The model under review builds one solid part; all positions refer to its coordinate system, in mm. A direction names the side the tool comes from. Coordinates: 2 decimals unless noted, no trailing zeros. Loops run counter-clockwise (first coordinate to the right, second up) from the corner with the lowest first, then second, coordinate; pieces in that order, holes last. Notation, with made-up numbers: (79, 12.5) - (103, 12.5) arc R5 cw to (103, 21.5) - close; hole circle Ø7 at (-33.5, -10). An arc over 180 degrees is marked (long way). One line per item, written item: value. Start each with the question number.
1. To check wall thickness, follow line 1 (Z direction, x = -60.75, y = 7.5); line 2 (X direction, y = 1.5, z = 12.75); line 3 (Z direction, x = -57, y = 10). State the ranges of each line that lie inside material, in increasing order.
2. We need section A-A, the plane z = 1.75. Give the boundary of the cut face in (x, y), then the cut area to 3 significant figures.
3. Mouldability with a two-part tool opening along X and no side actions: class faces 1 (the face through (-59, 1, 8.75)), 2 (the face through (-63, 5, 10)), 3 (the face through (-55, 1, 4)) as +X half, -X half, draft (parallel to the pull), parting line (faces both ways), or undercut.
4. We need section C-C, the plane y = 6.75. Give the boundary of the cut face in (x, z), then the cut area to 3 significant figures.
5. We need section B-B, the plane z = 10. Give the boundary of the cut face in (x, y).
6. We need section D-D, the plane x = -36.5. Give the boundary of the cut face in (y, z), then the cut area to 3 significant figures.
7. Insertion check: P1, Ø2, axis at x = -5.5, y = 1, coming from the -Z side; P2, Ø2.5, axis at y = 6, z = 10, coming from the +X side; P3, Ø3, axis at x = -52.5, z = 9.5, coming from the -Y side. Each pin has a flat end and moves straight along its axis. Give the tip position at first contact, or say it passes through.
8. For faces 4 (the face through (-9, 1, 11.25)), 5 (the face through (-37.1, 3.5, 9.9)), 6 (the face through (-8, 0, 4)), 7 (the face through (-55, 1, 16)), list the 3-axis set-ups (+Z, -Z, +X, -X, +Y, -Y) from which the entire face can be reached by the end or side of a thin tool; tool diameter is ignored.
Autodesk Inventor part; units mm, degrees
ref_plane "YZ Plane" through (0, 0, 0) normal (1, 0, 0) x (0, 1, 0)
ref_plane "XZ Plane" through (0, 0, 0) normal (0, 1, 0) x (-1, 0, 0)
ref_plane "XY Plane" through (0, 0, 0) normal (0, 0, 1) x (1, 0, 0)
sketch "Sketch1" plane through (0, 0, 0) normal (0, 0, 1) x (1, 0, 0)
  line L0 (0, 0) -> (0, 4)
  line L1 (0, 0) -> (-63, 0)
  line L2 (-63, 0) -> (-63, 12)
  line L3 (-63, 12) -> (0, 4)
  dimension "d0" = 4
  dimension "d1" = 63
  dimension "d2" = 12
extrude "Extrusion1" add sketch "Sketch1" along normal blind 20
sketch "Sketch2" plane through (-63, 0, 0) normal (-1, 0, 0) x (0, 0, 1)
  line L0 (0, 0) -> (20, 0)
  line L1 (10, 0) -> (8.75, 0)
  line L2 (8.75, 0) -> (8.75, 2)
  line L3 (8.75, 2) -> (10, 2)
  line L4 (10, 2) -> (10, 0)
  line L5 (10, 0) -> (11.25, 0)
  line L6 (11.25, 0) -> (11.25, 2)
  line L7 (11.25, 2) -> (10, 2)
  line L8 (10, 2) -> (10, 0)
  line L9 (0, 0) -> (20, 0)
  dimension "d5" = 1.25
  dimension "d6" = 2
  dimension "d7" = 1.25
extrude "Extrusion2" cut sketch "Sketch2" against normal through all
ref_plane "Work Plane1" through (-60, 0, 0) normal (-1, 0, 0) x (0, 0, 1)
sketch "Sketch3" plane through (-60, 0, 0) normal (-1, 0, 0) x (0, 0, 1)
  line L0 (0, 12) -> (20, 12)
  circle A0 centre (10, 7.5) radius 4
  line L1 (6, 7.5) -> (14, 7.5)
  line L2 (14, 7.5) -> (14, 12)
  line L3 (14, 12) -> (6, 12)
  line L4 (6, 12) -> (6, 7.5)
  line L5 (20, 4) -> (20, 12)
  point P0 (0, 0)
  dimension "d12" = 8
  dimension "d11" = 4.5
  dimension "d27" = 10
extrude "Extrusion3" cut sketch "Sketch3" against normal through all
hole "Hole1" at (-60, 7.5, 10) direction (-1, 0, 0) diameter 4.5 end through all
sketch "Sketch4" plane through (-63, 0, 0) normal (0, -1, 0) x (1, 0, 0)
  point P0 (63, 0)
sketch "Sketch5" plane through (-63, 0, 0) normal (0, -1, 0) x (1, 0, 0)
  line L0 (46, 20) -> (46, 0)
  line L1 (8, 0) -> (46, 0)
  line L2 (46, 0) -> (46, 20)
  line L3 (46, 20) -> (8, 20)
  line L4 (8, 20) -> (8, 0)
  point P0 (0, 0)
  dimension "d23" = 46
  dimension "d26" = 8
extrude "Extrusion4" cut sketch "Sketch5" against normal up to surface (2 mm away)
properties part number "support_lcd_v2"
Findings below:
1. line 1: 0 to 7.75, 12.25 to 20
1. line 2: -63 to -55, -17 to 0
1. line 3: 0 to 6, 14 to 20
2. outline: (-63, 0) - (-55, 0) - (-55, 2) - (-17, 2) - (-17, 0) - (0, 0) - (0, 4) - (-63, 12) - close
2. area: 428 mm2
3. face 1: draft
3. face 2: -X half
3. face 3: undercut
4. outline: (-63, 0) - (-21.66, 0) - (-21.66, 6.07) - (-60, 6.07) - (-60, 7.88) - (-63, 7.88) - close; (-63, 12.12) - (-60, 12.12) - (-60, 13.93) - (-21.66, 13.93) - (-21.66, 20) - (-63, 20) - close
4. area: 513 mm2
5. outline: (-63, 2) - (0, 2) - (0, 3.5) - (-60, 3.5) - (-60, 5.25) - (-63, 5.25) - close; (-63, 9.75) - (-60, 9.75) - (-60, 11.62) - (-63, 12) - close
6. outline: (2, 0) - (8.63, 0) - (8.63, 6) - (7.5, 6) arc R4 cw to (7.5, 14) - (8.63, 14) - (8.63, 20) - (2, 20) - close
6. area: 98.5 mm2
7. P1: z = 0
7. P2: x = -60
7. P3: y = 2
8. face 4: +X, -X, -Y
8. face 5: +X, +Y
8. face 6: +Z, -Z, +X, -X, -Y
8. face 7: +Z, -Z, -Y
